Part print with two shaded views. Sizes in mm from the minimum x, y, z corner. A direction names the side the tool comes from. Coordinates: 2 decimals unless noted, no trailing zeros. Write each loop counter-clockwise with the first axis right and the second up, starting at its lowest first coordinate (ties: lowest second). Pieces come first, ordered by that corner, then holes.
Q1. Pin check, flat tip, straight feed: P1, Ø5, axis at x = 112, y = 58, coming from the +Z side. Stop position of the tip, or through.
Q2. Band-saw the part on C-C, the plane x = 12.5. Write the cut outline in (y, z).
Q3. Drill centre lines: probe 1 along X at (y, z) = (53, 14.25); probe 2 along Z at (x, y) = (2.5, 42.5); probe 3 along Y at (x, z) = (93, 11.25). Where is each one in solid material? Low to high.
Q4. Which spindle directions (+Z, -Z, +X, -X, +Y, -Y) get a long thin tool onto all of the face, cutting with end or side? Do the marked faces 1 and 2. Say none if no direction does.
Q5. Pull direction X, two halves, no side cores. Call the marked faces 3, 4, 5 and 6: released by +X, released by -X, zero draft, split by the parting line, or undercut.
Q6. Band-saw the part on B-B, the plane z = 16.25. Write the cut outline in (x, y), plus the area to 3 significant figures.
Q7. Band-saw the part on A-A, the plane y = 32.5. Write the cut outline in (x, z).
Q8. Band-saw the part on D-D, the plane y = 49. Write the cut outline in (x, z), plus the area to 3 significant figures.
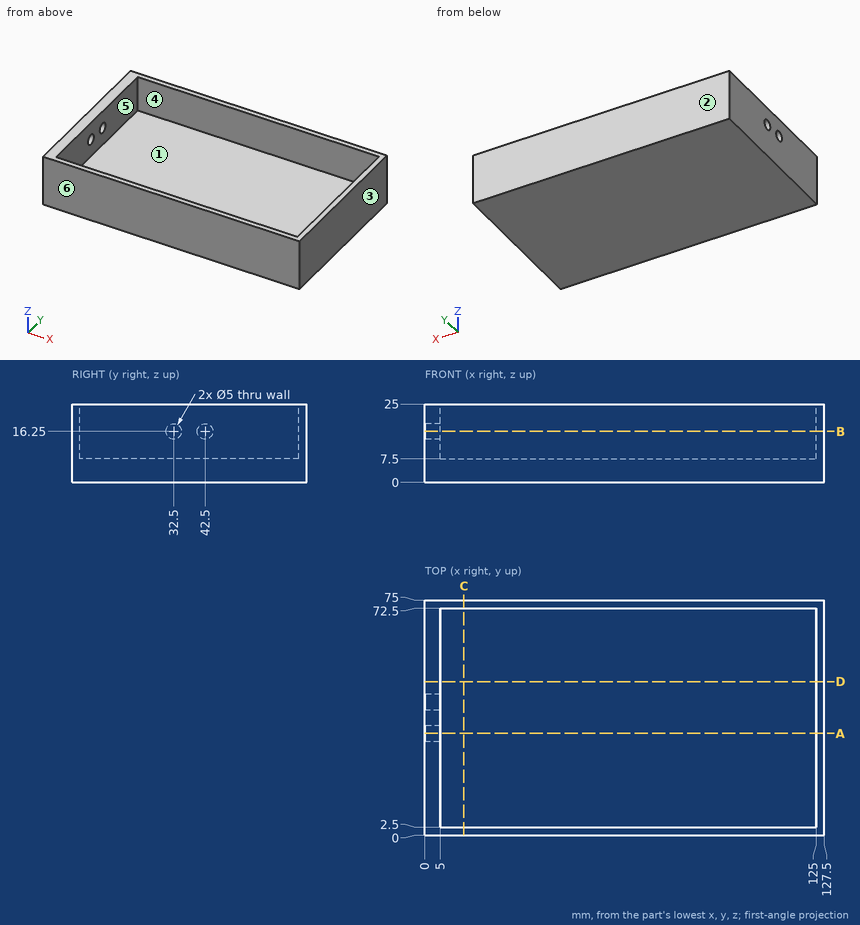
Answer sheet:
1. P1: stops at z = 7.5
2. outline: (0, 0) - (75, 0) - (75, 25) - (72.5, 25) - (72.5, 7.5) - (2.5, 7.5) - (2.5, 25) - (0, 25) - close
3. probe 1: x = 0 to 5, 125 to 127.5
3. probe 2: z = 0 to 13.75, 18.75 to 25
3. probe 3: y = 0 to 2.5, 72.5 to 75
4. face 1: +Z
4. face 2: +Z, -Z, +X, -X, +Y
5. face 3: released by +X
5. face 4: undercut
5. face 5: undercut
5. face 6: zero draft
6. outline: (0, 0) - (127.5, 0) - (127.5, 75) - (0, 75) - (0, 45) - (5, 45) - (5, 72.5) - (125, 72.5) - (125, 2.5) - (5, 2.5) - (5, 30) - (0, 30) - close; (0, 35) - (5, 35) - (5, 40) - (0, 40) - close
6. area: 1,110 mm2
7. outline: (0, 0) - (127.5, 0) - (127.5, 25) - (125, 25) - (125, 7.5) - (5, 7.5) - (5, 13.75) - (0, 13.75) - close; (0, 18.75) - (5, 18.75) - (5, 25) - (0, 25) - close
8. outline: (0, 0) - (127.5, 0) - (127.5, 25) - (125, 25) - (125, 7.5) - (5, 7.5) - (5, 25) - (0, 25) - close
8. area: 1,090 mm2
